Work out the finished part from the listing and answer in its coordinate system (mm). Face numbers are marked on the shaded views. A direction names the side the tool comes from. Coordinates: 2 decimals unless noted, no trailing zeros. Order: outer loops, then holes, each group sorted by start corner. A loop starts at its lowest first (then second) coordinate and runs counter-clockwise, first axis right, second up. Notation, with made-up numbers: (43, 37.5) -> (59, 37.5) arc R24 ccw to (59, 64.5) -> close; hole circle Ø4 at (-4, 1). An arc over 180 degrees is marked (long way). Use one line per item in the form item = value.
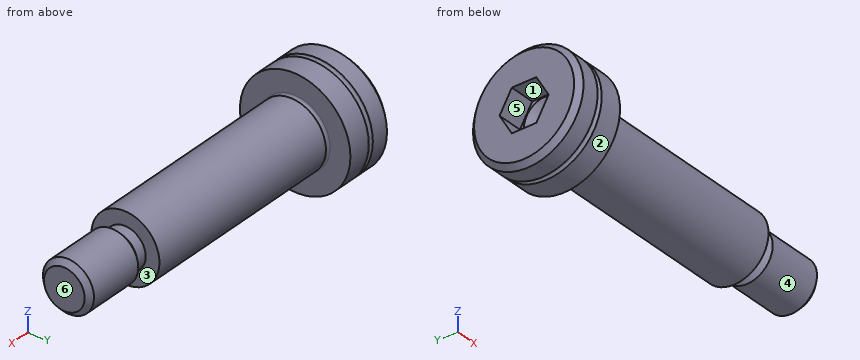
from build123d import *

# Parameters (mm, degrees)
SKETCH2_R           = 3.84
BOSS_EXTRUDE1_DEPTH = 0.387623957
SKETCH3_R           = 3.84
BOSS_EXTRUDE2_DEPTH = 0.092376043
BOSS_EXTRUDE2_TAPER = -60.000000004
SKETCH4_R           = 4
BOSS_EXTRUDE3_DEPTH = 24.52
SKETCH5_R           = 2.3865
BOSS_EXTRUDE4_DEPTH = 1.25
SKETCH6_R           = 2.3865
BOSS_EXTRUDE5_DEPTH = 0.6135
BOSS_EXTRUDE5_TAPER = -45
SKETCH7_R           = 3
BOSS_EXTRUDE6_DEPTH = 7.1365
CUT_EXTRUDE1_DEPTH  = 3
CHAMFER1_SIZE       = 0.6135
FILLET1_R           = 0.261


with BuildPart() as part:
    # Sketch1 → Revolve1 (revolve)
    with BuildSketch(Plane(origin=(0, 0, 0), x_dir=(-1, 0, 0), z_dir=(0, 0, -1))):
        with BuildLine():
            Line((0, 6.5), (0, 0))
            Line((0, 0), (6, 0))
            Line((6, 0), (6, 6.5))
            Line((6, 6.5), (3.3, 6.5))
            ThreePointArc((3.3, 6.5), (3, 6.2), (2.7, 6.5))
            Line((2.7, 6.5), (0, 6.5))
        make_face()
    revolve(axis=Axis((0, 0, 0), (-1, 0, 0)))

    # Sketch2 → Boss-Extrude1 (add)
    with BuildSketch(Plane(origin=(0, 0, 0), x_dir=(0, 0, -1), z_dir=(1, 0, 0))):
        Circle(SKETCH2_R)
    extrude(amount=BOSS_EXTRUDE1_DEPTH)

    # Sketch3 → Boss-Extrude2 (add)
    with BuildSketch(Plane(origin=(0.387623957, 0, 0), x_dir=(0, 0, -1), z_dir=(1, 0, 0))):
        Circle(SKETCH3_R)
    extrude(amount=BOSS_EXTRUDE2_DEPTH, taper=BOSS_EXTRUDE2_TAPER)

    # Sketch4 → Boss-Extrude3 (add)
    with BuildSketch(Plane(origin=(0.48, 0, 0), x_dir=(0, 0, -1), z_dir=(1, 0, 0))):
        Circle(SKETCH4_R)
    extrude(amount=BOSS_EXTRUDE3_DEPTH)

    # Sketch5 → Boss-Extrude4 (add)
    with BuildSketch(Plane(origin=(25, 0, 0), x_dir=(0, 0, -1), z_dir=(1, 0, 0))):
        Circle(SKETCH5_R)
    extrude(amount=BOSS_EXTRUDE4_DEPTH)

    # Sketch6 → Boss-Extrude5 (add)
    with BuildSketch(Plane(origin=(26.25, 0, 0), x_dir=(0, 0, -1), z_dir=(1, 0, 0))):
        Circle(SKETCH6_R)
    extrude(amount=BOSS_EXTRUDE5_DEPTH, taper=BOSS_EXTRUDE5_TAPER)

    # Sketch7 → Boss-Extrude6 (add)
    with BuildSketch(Plane(origin=(26.8635, 0, 0), x_dir=(0, 0, -1), z_dir=(1, 0, 0))):
        Circle(SKETCH7_R)
    extrude(amount=BOSS_EXTRUDE6_DEPTH)

    # Sketch8 → Cut-Extrude1 (cut)
    with BuildSketch(Plane.ZY.offset(6)):
        Polygon((2.5, -1.443375673), (2.5, 1.443375673), (0, 2.886751346), (-2.5, 1.443375673), (-2.5, -1.443375673), (0, -2.886751346), align=None)
    extrude(amount=-CUT_EXTRUDE1_DEPTH, mode=Mode.SUBTRACT)

    # Sketch9 → Cut-Revolve1 (revolve, cut)
    with BuildSketch(Plane.XY):
        Polygon((-3, 2.4), (-3, 0), (-1.614359354, 0), align=None)
    revolve(axis=Axis((-3, 0, 0), (1, 0, 0)), mode=Mode.SUBTRACT)

    # Chamfer1
    chamfer1_edges = [part.edges().sort_by_distance(p)[0] for p in [
        (34, 0, 3),
        (-6, -6.5, 0),
    ]]
    chamfer(chamfer1_edges, length=CHAMFER1_SIZE)

    # Fillet1
    fillet1_edges = [part.edges().sort_by_distance(p)[0] for p in [
        (0, 0, 3.84),
    ]]
    fillet(fillet1_edges, radius=FILLET1_R)


solid = part.part
(1) Which of the six approach directions +Z, -Z, +X, -X, +Y, -Y give full straight-line access (tool end or side, diameter ignored) to the marked faces 4, 5 and 6?
Data:
face_4 = +X
face_5 = -X
face_6 = +Z, -Z, +X, +Y, -Y
(2) Straight lines are drawn through the part: line 1 along X through (y, z) = (-4.75, 3.25); line 2 along Z through (x, y) = (3.5, -0.25). For each, find the intervals that lie inside material, in ascending order.
Data:
line_1 = -6 to 0
line_2 = -3.99 to 3.99
(3) The mould has two halves that part along Y. Classify the marked faces 1, 2 and 3: released by +Y, released by -Y, zero draft, split by the parting line, or undercut.
Data:
face_1 = undercut
face_2 = split by the parting line
face_3 = zero draft
(4) Section A-A on x = 23 is taken. Write down the section's boundary in (y, z), plus the area to 3 significant figures.
Data:
outline = circle Ø8 at (0, 0)
area = 50.3 mm²
(5) Each of these flat-tipped pins is pushed along its axis until it touches: P1, Ø4, axis at x = 1, y = 5, coming from the -Z side; P2, Ø1.5, axis at y = 2, z = -5, coming from the +X side; P3, Ø1, axis at x = 2.5, y = 2, coming from the +Z side. Where does it stop, or does it pass through?
Data:
P1 = -5.62
P2 = 0
P3 = 3.71
